Could you check a few things on this model? Use its own coordinates, in mm. A direction names the side the tool comes from. Coordinates: 2 decimals unless noted, no trailing zeros. Loops run counter-clockwise (first coordinate to the right, second up) from the corner with the lowest first, then second, coordinate; pieces in that order, holes last. Notation, with made-up numbers: (61.25, 18.25) - (118.25, 18.25) arc R18 cw to (118.25, 47.25) - close; hole circle Ø2 at (63, 46.25). An arc over 180 degrees is marked (long way). One line per item, written item: value. Start each with the question number.
(1) If we mould it in two halves opening along X, with no side actions, what happens to faces 1 (the face through (2.995, 1.662, 9.618)), 2 (the face through (0, 0, 0)), 3 (the face through (0, 0, 7))? For each: pulls with the +X half, pulls with the -X half, needs draft (parallel to the pull), parting line crosses it, or undercut.
(2) If we section it at B-B on z = 1.5: Write out the boundary of the cut face in (x, y).
(3) If we section it at A-A on z = 17: Write out the boundary of the cut face in (x, y), then the cut area to 3 significant figures.
(4) On a 3-axis mill with a long thin cutter (end or side, diameter ignored), from which of +Z, -Z, +X, -X, +Y, -Y can I reach the whole of each face in a straight line? I mean faces 4 (the face through (0, 1.5, 11)), 5 (the face through (2.89, -1.67, 19.41)). Say none if no direction works.
(5) If we section it at C-C on z = 7.25: Write out the boundary of the cut face in (x, y).
(6) I'm going to push flat-ended pins straight in: P1, Ø1, axis at x = 0, y = -1, coming from the +Z side; P2, Ø3, axis at y = 1.5, z = 16, coming from the +X side; P3, Ø3, axis at x = 0, z = 10, coming from the -Y side. Where does each tip first touch, or does it pass through?
(7) If I drill on line 1 along Y through (x, z) = (1.5, 16.25); line 2 along Z through (x, y) = (0.5, -1.25); line 3 along Y through (x, z) = (-0.75, 16.75), over which ranges is the centre line in solid material (lowest first)? Write a range as from..to.
```python
from build123d import *
from build123d.topology import SkipClean

# Parameters (mm, degrees)
EXTRUDE_1_DEPTH     = 19.5
CUT_EXTRUDE_1_DEPTH = 12.5
SKETCH_3_R          = 2
CUT_EXTRUDE_2_DEPTH = 4
FILLET_1_R          = 0.3
FILLET_2_R          = 0.2


with BuildPart() as part:
    # Эскиз1 → Бобышка-Вытянуть1 (new body)
    with BuildSketch(Plane.XY):
        Polygon((2.008322, 3.406975), (-1.946366, 3.442745), (-3.954688, 0.03577), (-2.008322, -3.406975), (1.946366, -3.442745), (3.954688, -0.03577), align=None)
    extrude(amount=EXTRUDE_1_DEPTH)

    # Эскиз2 → Вырез-Вытянуть1 (cut)
    with BuildSketch(Plane.XY.offset(19.5)):
        with BuildLine():
            Line((-1.322876, 1.5), (1.322876, 1.5))
            ThreePointArc((1.322876, 1.5), (0, -2), (-1.322876, 1.5))
        make_face()
    extrude(amount=-CUT_EXTRUDE_1_DEPTH, mode=Mode.SUBTRACT)

    # Эскиз3 → Вырез-Вытянуть2 (cut)
    with SkipClean():  # the faces are left unmerged after this step: merging them gives an invalid solid
        with BuildSketch(Plane.XY.offset(19.5)):
            Circle(SKETCH_3_R)
        extrude(amount=-CUT_EXTRUDE_2_DEPTH, mode=Mode.SUBTRACT)

    # Скругление1
    fillet_1_edges = [part.edges().sort_by_distance(p)[0] for p in [
        (-2.950527, 1.739258, 19.5),
        (-2.981505, -1.685602, 19.5),
        (-0.030978, -3.42486, 19.5),
        (2.950527, -1.739258, 19.5),
        (-0.822876, -1.822876, 19.5),
        (2.981505, 1.685602, 19.5),
        (2.950527, -1.739258, 0),
        (-0.030978, -3.42486, 0),
        (-2.981505, -1.685602, 0),
        (0.030978, 3.42486, 19.5),
        (-2.950527, 1.739258, 0),
        (0.030978, 3.42486, 0),
        (2.981505, 1.685602, 0),
    ]]
    fillet(fillet_1_edges, radius=FILLET_1_R)

    # Скругление2
    # the kernel refuses this fillet: 0.2 mm, written as the material it takes off along each edge
    with BuildSketch(Plane(origin=(1.822876, 1.5, 15.5), x_dir=(0, 1, 0), z_dir=(-1, 0, 0))) as fillet_2_piece_1_section:
        with BuildLine():
            CenterArc((FILLET_2_R, FILLET_2_R), FILLET_2_R, 180, 90)
            Line((0, FILLET_2_R), (0, 0))
            Line((0, 0), (FILLET_2_R, 0))
        make_face()
    fillet_2_piece_1 = extrude(amount=3.645751, mode=Mode.PRIVATE)
    fillet_2_piece_1 = fillet_2_piece_1 & Plane(origin=(0, 0, 15.453639), x_dir=(0.6614378277661478, 0.75, 0), z_dir=(0, 0, 1)) * Cylinder(2, 9, mode=Mode.PRIVATE)
    add(fillet_2_piece_1, mode=Mode.SUBTRACT)


solid = part.part
```
Values:
1. face 1: pulls with the +X half
1. face 2: needs draft
1. face 3: undercut
2. outline: (-3.95, 0.04) - (-2.01, -3.41) - (1.95, -3.44) - (3.95, -0.04) - (2.01, 3.41) - (-1.95, 3.44) - close
3. outline: (-3.95, 0.04) - (-2.01, -3.41) - (1.95, -3.44) - (3.95, -0.04) - (2.01, 3.41) - (-1.95, 3.44) - close; hole circle Ø4 at (0, 0)
3. area: 28.1 mm2
4. face 4: +Z
4. face 5: +Z, +X, -Y
5. outline: (-3.95, 0.04) - (-2.01, -3.41) - (1.95, -3.44) - (3.95, -0.04) - (2.01, 3.41) - (-1.95, 3.44) - close; hole (-1.32, 1.5) arc R2 ccw (long way) to (1.32, 1.5) - close
6. P1: stops at z = 7
6. P2: stops at x = 3.93
6. P3: stops at y = -3.44
7. line 1: y = -3.44..-1.32, 1.32..3.41
7. line 2: z = 0..7
7. line 3: y = -3.42..-1.85, 1.85..3.43
